from build123d import *

# Parameters (mm, degrees)
SKETCH_1_R      = 5
EXTRUDE_1_DEPTH = 3
FILLET_1_R      = 5
FILLET_2_R      = 5
FILLET_3_R      = 5


with BuildPart() as part:
    # 草图1 → 凸台-拉伸1 (new body)
    with BuildSketch(Plane.XY):
        with BuildLine():
            Line((101.056239558, 66.72819932), (0, 53))
            Line((0, 53), (-101.056239558, 66.72819932))
            Line((-101.056239558, 66.72819932), (-103.05702305, 67))
            ThreePointArc((-103.05702305, 67), (-110.280675742, 61.517137029), (-106.942649005, 53.085024478))
            Line((-106.942649005, 53.085024478), (-5.180834606, -8.553300696))
            ThreePointArc((-5.180834606, -8.553300696), (-3.881694774, -9.215880082), (-2.5, -9.682458366))
            ThreePointArc((-2.5, -9.682458366), (0, -10), (2.5, -9.682458366))
            ThreePointArc((2.5, -9.682458366), (3.881694774, -9.215880082), (5.180834606, -8.553300696))
            Line((5.180834606, -8.553300696), (106.942649005, 53.085024478))
            ThreePointArc((106.942649005, 53.085024478), (110.280675742, 61.517137029), (103.05702305, 67))
            Line((103.05702305, 67), (101.056239558, 66.72819932))
        make_face()
        Circle(SKETCH_1_R, mode=Mode.SUBTRACT)
        with BuildLine():
            Line((-38.470197272, 17.456153435), (-2.5, 47.638732699))
            Line((-2.5, 47.638732699), (-2.5, 9.682458366))
            ThreePointArc((-2.5, 9.682458366), (-7.840929555, 6.206434058), (-9.997792991, 0.210084034))
            Line((-9.997792991, 0.210084034), (-38.470197272, 17.456153435))
        make_face(mode=Mode.SUBTRACT)
        with BuildLine():
            Line((38.470197272, 17.456153435), (9.997792991, 0.210084034))
            ThreePointArc((9.997792991, 0.210084034), (7.840929555, 6.206434058), (2.5, 9.682458366))
            Line((2.5, 9.682458366), (2.5, 47.638732699))
            Line((2.5, 47.638732699), (38.470197272, 17.456153435))
        make_face(mode=Mode.SUBTRACT)
        Polygon((-76.992375251, 58.413267417), (-46.919815599, 22.574186413), (-91.163166243, 49.372903102), (-79.915961764, 58.810428231), align=None, mode=Mode.SUBTRACT)
        Polygon((-69.625606174, 57.412513038), (-8.52297152, 49.111895964), (-40.292213402, 22.454336819), align=None, mode=Mode.SUBTRACT)
        with BuildLine():
            Line((-95.680736217, 52.109248249), (-98.304134778, 53.698271544))
            ThreePointArc((-98.304134778, 53.698271544), (-95.998027486, 56.966113336), (-95.699425849, 60.954566405))
            Line((-95.699425849, 60.954566405), (-86.610723734, 59.719892378))
            Line((-86.610723734, 59.719892378), (-95.680736217, 52.109248249))
        make_face(mode=Mode.SUBTRACT)
        with BuildLine():
            ThreePointArc((-103.304614869, 61.987709447), (-102.720496256, 61.977246398), (-102.154754916, 61.831504281))
            ThreePointArc((-102.154754916, 61.831504281), (-100.994782723, 60.913210824), (-100.55702305, 59.5))
            ThreePointArc((-100.55702305, 59.5), (-104.73497127, 57.646762354), (-103.304614869, 61.987709447))
        make_face(mode=Mode.SUBTRACT)
        Polygon((40.292213402, 22.454336819), (8.52297152, 49.111895964), (69.625606174, 57.412513038), align=None, mode=Mode.SUBTRACT)
        Polygon((91.163166243, 49.372903102), (46.919815599, 22.574186413), (76.992375251, 58.413267417), (79.915961764, 58.810428231), align=None, mode=Mode.SUBTRACT)
        with BuildLine():
            Line((95.680736217, 52.109248249), (86.610723734, 59.719892378))
            Line((86.610723734, 59.719892378), (95.699425849, 60.954566405))
            ThreePointArc((95.699425849, 60.954566405), (95.998027486, 56.966113336), (98.304134778, 53.698271544))
            Line((98.304134778, 53.698271544), (95.680736217, 52.109248249))
        make_face(mode=Mode.SUBTRACT)
        with BuildLine():
            ThreePointArc((105.55702305, 59.5), (101.643812227, 57.437759673), (102.154754916, 61.831504281))
            ThreePointArc((102.154754916, 61.831504281), (102.720496256, 61.977246398), (103.304614869, 61.987709447))
            ThreePointArc((103.304614869, 61.987709447), (104.910260696, 61.177948219), (105.55702305, 59.5))
        make_face(mode=Mode.SUBTRACT)
    extrude(amount=EXTRUDE_1_DEPTH)

    # 圆角1
    # the kernel refuses this fillet: 5 mm, written as the material it adds along each edge
    with BuildSketch(Plane(origin=(76.992375251, 58.413267417, 0), x_dir=(0.9908985592379703, 0.1346107176272178, 0), z_dir=(0, 0, 1))) as fillet_1_piece_1:
        with BuildLine():
            CenterArc((FILLET_1_R * 0.386508582556, -FILLET_1_R), FILLET_1_R, 90, 42.263889815)
            Line((-FILLET_1_R * 0.286037651021, -FILLET_1_R * 0.259944891443), (0, 0))
            Line((0, 0), (FILLET_1_R * 0.386508582556, 0))
        make_face()
    extrude(amount=3)
    with BuildSketch(Plane(origin=(79.915961764, 58.810428231, 0), x_dir=(0.7660444431189772, -0.6427876096865403, 0), z_dir=(0, 0, 1))) as fillet_1_piece_2:
        with BuildLine():
            CenterArc((FILLET_1_R * 0.442472138408, -FILLET_1_R), FILLET_1_R, 90, 47.736110185)
            Line((-FILLET_1_R * 0.297582970149, -FILLET_1_R * 0.327453766423), (0, 0))
            Line((0, 0), (FILLET_1_R * 0.442472138408, 0))
        make_face()
    extrude(amount=3)

    # 圆角2
    # the kernel refuses this fillet: 5 mm, written as the material it adds along each edge
    with BuildSketch(Plane(origin=(-79.915961764, 58.810428231, 0), x_dir=(0.9908985592379704, -0.13461071762721746, 0), z_dir=(0, 0, 1))) as fillet_2_piece_1:
        with BuildLine():
            CenterArc((FILLET_2_R * 0.442472138408, -FILLET_2_R), FILLET_2_R, 90, 47.736110185)
            Line((-FILLET_2_R * 0.297582970149, -FILLET_2_R * 0.327453766423), (0, 0))
            Line((0, 0), (FILLET_2_R * 0.442472138408, 0))
        make_face()
    extrude(amount=3)
    with BuildSketch(Plane(origin=(-76.992375251, 58.413267417, 0), x_dir=(0.642787609686538, -0.7660444431189791, 0), z_dir=(0, 0, 1))) as fillet_2_piece_2:
        with BuildLine():
            CenterArc((FILLET_2_R * 0.386508582556, -FILLET_2_R), FILLET_2_R, 90, 42.263889815)
            Line((-FILLET_2_R * 0.286037651021, -FILLET_2_R * 0.259944891443), (0, 0))
            Line((0, 0), (FILLET_2_R * 0.386508582556, 0))
        make_face()
    extrude(amount=3)

    # 圆角3
    fillet_3_edges = [part.edges().sort_by_distance(p)[0] for p in [
        (-2.5, 9.682458366, 1.5),
        (2.5, 9.682458366, 1.5),
    ]]
    fillet(fillet_3_edges, radius=FILLET_3_R)


solid = part.part
For this review, take the finished solid that the model builds, in its own axes (mm). A direction names the side the tool comes from. Give positions to 0.01 mm unless a question says otherwise; leave off trailing zeros. Order: outer loops, then holes, each group sorted by start corner. A loop starts at its lowest first (then second) coordinate and runs counter-clockwise, first axis right, second up. Notation, with made-up numbers: M 33.25,55 L 51.25,55 A20 cw 51.25,76 Z; hole C 25.5,59.5 d4. An arc over 180 degrees is marked long. Answer in a Markdown table with one row per item. Add a question column.
(1) Consider section B-B on y = 28. State the section outline as (x, z) points.
(2) Consider section D-D on x = 26. State the section outline as (y, z) points.
(3) Consider section C-C on z = 0.55. Give the number of separate pieces and of enclosed holes in the cut face, and give its area (3 significant figures).
(4) Mouldability with a two-part tool opening along Y and no side actions: class faces 3 (the face through (1, 39, 3)), 4 (the face through (86.32, 53.437, 1.479)), 5 (the face through (-110.243, 61.648, 1.479)), 6 (the face through (38.647, 53.204, 1.479)) as +Y half, -Y half, draft (parallel to the pull), parting line (faces both ways), or undercut.
(5) Consider section A-A on x = -66. State the section outline as (y, z) points.
(6) For faces 1 (the face through (-68.732, 35.786, 1.479)), 2 (the face through (1, 39, 0)), list the 3-axis set-ups (+Z, -Z, +X, -X, +Y, -Y) from which the entire face can be reached by the end or side of a thin tool; tool diameter is ignored.
(7) Wall thickness on probe 1 along Y at (x, z) = (-60.5, 1.95); probe 2 along Y at (x, z) = (30.5, 0.55); probe 3 along X at (y, z) = (14.5, 2.3): over which ranges is each line inside the solid? List them lowest first. Write a range as [from, to].
(8) For pin 1 (0.9 mm diameter, centred on y = 27, z = 1.5, fed in from -X); pin 2 (0.9 mm diameter, centred on y = 30, z = 1.5, fed in from +X); pin 3 (1.5 mm diameter, centred on x = -44.5, y = 25.5, fed in from -Z); pin 4 (1 mm diameter, centred on y = 19.5, z = 1, fed in from +X), all flat-tipped, find the tip position at first contact; note any pin that passes through.
Evaluation:
| question | item | result |
|---|---|---|
| 1 | outline | M -65.53,0 L -55.88,0 L -55.88,3 L -65.53,3 Z; M -51.47,0 L -44.95,0 L -44.95,3 L -51.47,3 Z; M -33.68,0 L -25.9,0 L -25.9,3 L -33.68,3 Z; M -2.5,0 L 2.5,0 L 2.5,3 L -2.5,3 Z; M 25.9,0 L 33.68,0 L 33.68,3 L 25.9,3 Z; M 44.95,0 L 51.47,0 L 51.47,3 L 44.95,3 Z; M 55.88,0 L 65.53,0 L 65.53,3 L 55.88,3 Z |
| 2 | outline | M 4.06,0 L 9.9,0 L 9.9,3 L 4.06,3 Z; M 27.92,0 L 34.45,0 L 34.45,3 L 27.92,3 Z; M 51.49,0 L 56.53,0 L 56.53,3 L 51.49,3 Z |
| 3 | separate pieces | 1 |
| 3 | enclosed holes | 11 |
| 3 | area | 3,880 mm^2 |
| 4 | face 3 | draft |
| 4 | face 4 | undercut |
| 4 | face 5 | parting line |
| 4 | face 6 | undercut |
| 5 | outline | M 28.29,0 L 34.13,0 L 34.13,3 L 28.29,3 Z; M 45.31,0 L 53.09,0 L 53.09,3 L 45.31,3 Z; M 56.92,0 L 61.97,0 L 61.97,3 L 56.92,3 Z |
| 6 | face 1 | +Z, -Z |
| 6 | face 2 | -Z, +X, -X, +Y, -Y |
| 7 | probe 1 | y = [24.95, 30.8], [38.76, 46.54], [56.17, 61.22] |
| 7 | probe 2 | y = [6.78, 12.63], [24.14, 30.67], [52.1, 57.14] |
| 7 | probe 3 | x = [-43.24, -33.59], [-2.5, 2.5], [33.59, 43.24] |
| 8 | pin 1 | stops at x = -64.62 |
| 8 | pin 2 | stops at x = 69.57 |
| 8 | pin 3 | stops at z = 0 |
| 8 | pin 4 | stops at x = 52.32 |
